Geometry check sheet. Reference: the model listing, model coordinates, mm. Face numbers are marked on the shaded views. A direction names the side the tool comes from. Coordinates: 2 decimals unless noted, no trailing zeros. Write each loop counter-clockwise with the first axis right and the second up, starting at its lowest first coordinate (ties: lowest second). Pieces come first, ordered by that corner, then holes. Notation, with made-up numbers: (58.25, -13.5) -> (69.25, -13.5) arc R8 ccw to (69.25, -0.5) -> close; hole circle Ø9 at (0.5, -5.5). An arc over 180 degrees is marked (long way). Answer as CSV lines item,"result".
```python
from build123d import *

# Parameters (mm, degrees)
F1_DEPTH = 58.674
F2_R     = 26.7576481094
F3_DEPTH = 36.068
F4_R     = 5.08
F5_DEPTH = 214.122


with BuildPart() as f1:
    # F0 (on Top) → F1 (new body)
    with BuildSketch(Plane.XY):
        Polygon((35.4626365006, 51.1673055589), (-35.2130606771, 50.5765117705), (-35.2130606771, -29.6294502914), (35.4626365006, -29.6294502914), align=None)
    extrude(amount=F1_DEPTH)

    # F2 (on face) → F3 (cut)
    with BuildSketch(Plane.XY.offset(58.674)):
        with Locations((0, 12.6274535432)):
            Circle(F2_R)
    extrude(amount=-F3_DEPTH, mode=Mode.SUBTRACT)

    # F4 (on face) → F5 (join)
    with BuildSketch(Plane.XY.offset(58.674)):
        with Locations((-22.9736331001, -13.1111371607)):
            Circle(F4_R)
        with Locations((-22.9736331001, 37.6888628393)):
            Circle(F4_R)
        with BuildLine():
            ThreePointArc((18.7894253284, 31.6781550573), (23.486962927, 32.2345703811), (25.6893701616, 36.4209602192))
            ThreePointArc((25.6893701616, 36.4209602192), (19.3290072561, 41.3369617275), (16.1747753466, 33.9429027488))
            ThreePointArc((16.1747753466, 33.9429027488), (17.5187357631, 32.852824482), (18.7894253284, 31.6781550573))
        make_face()
        with Locations((20.6093701616, -13.1111371607)):
            Circle(F4_R)
    extrude(amount=-F5_DEPTH)


solid = f1.part
```
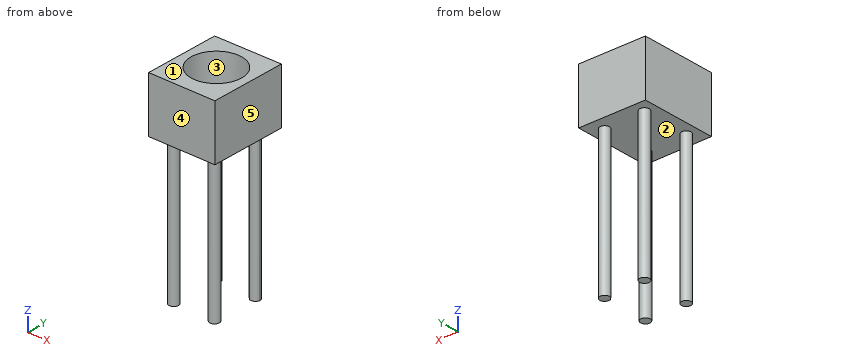
Item 1: Release check for a two-part mould opening along X. For the marked faces 3, 4 and 5 record: +X half, -X half, draft (parallel to the pull), parting line (faces both ways), or undercut.
Responses:
face 3,"undercut"
face 4,"draft"
face 5,"+X half"
Item 2: Set-up check for the marked faces 1 and 2: record each of +Z, -Z, +X, -X, +Y, -Y from which the full face is reachable in a straight line by a thin tool's end or side.
Responses:
face 1,"+Z, +X, -X, +Y, -Y"
face 2,"-Z"
Item 3: Cross-section at B-B, the plane x = 0. Record the cut outline in (y, z), plus the area to 3 significant figures.
Responses:
outline,"(-29.63, 0) -> (50.87, 0) -> (50.87, 58.67) -> (39.39, 58.67) -> (39.39, 22.61) -> (-14.13, 22.61) -> (-14.13, 58.67) -> (-29.63, 58.67) -> close"
area,"2,790 mm2"
Item 4: Cross-section at A-A, the plane y = 4. Record the cut outline in (x, z).
Responses:
outline,"(-35.21, 0) -> (35.46, 0) -> (35.46, 58.67) -> (25.33, 58.67) -> (25.33, 22.61) -> (-25.33, 22.61) -> (-25.33, 58.67) -> (-35.21, 58.67) -> close"
Item 5: Thickness scan on probe 1 along X at (y, z) = (-13, -46); probe 2 along Y at (x, z) = (21, -102); probe 3 along Z at (x, y) = (15.5, 46). Record the ranges inside material, lowest first.
Responses:
probe 1,"x = -28.05 to -17.89, 15.53 to 25.69"
probe 2,"y = -18.18 to -8.05, 31.36 to 41.49"
probe 3,"z = 0 to 58.67"
Item 6: Cross-section at C-C, the plane z = -113.5. Record the cut outline in (x, y).
Responses:
outline,"circle Ø10.16 at (-22.97, -13.11); circle Ø10.16 at (-22.97, 37.69); circle Ø10.16 at (20.61, -13.11); (16.17, 33.94) arc R26.76 cw to (18.79, 31.68) arc R5.08 ccw (long way) to start"
Item 7: Cross-section at D-D, the plane y = -23.5. Record the cut outline in (x, z), plus the area to 3 significant figures.
Responses:
outline,"(-35.21, 0) -> (35.46, 0) -> (35.46, 58.67) -> (-35.21, 58.67) -> close"
area,"4,150 mm2"
Item 8: Depth check by flat-ended pin: pin 1 Ø6 at (x, z) = (13, -112.5) entering from -Y; pin 2 Ø1.5 at (x, y) = (17.5, 16.5) entering from -Z; pin 3 Ø1.5 at (x, z) = (26.5, -78) entering from -Y; pin 4 Ø3 at (x, z) = (-27.5, -75) entering from +Y. Enter the tip coordinate at first touch or a pass-through.
Responses:
pin 1,"stops at y = -15.25"
pin 2,"stops at z = 0"
pin 3,"passes through"
pin 4,"stops at y = 41.77"
